Part print with two shaded views. Sizes in mm from the minimum x, y, z corner. Give positions to 0.01 mm unless a question says otherwise; leave off trailing zeros. Write each loop counter-clockwise with the first axis right and the second up, starting at its lowest first coordinate (ties: lowest second). Pieces come first, ordered by that corner, then holes. Notation, with made-up numbers: (44, 40) - (80, 40) arc R17 ccw to (80, 49) - close; hole circle Ø9 at (-9, 29.5). An arc over 180 degrees is marked (long way). Answer as a JSON object with one key per item and string values.
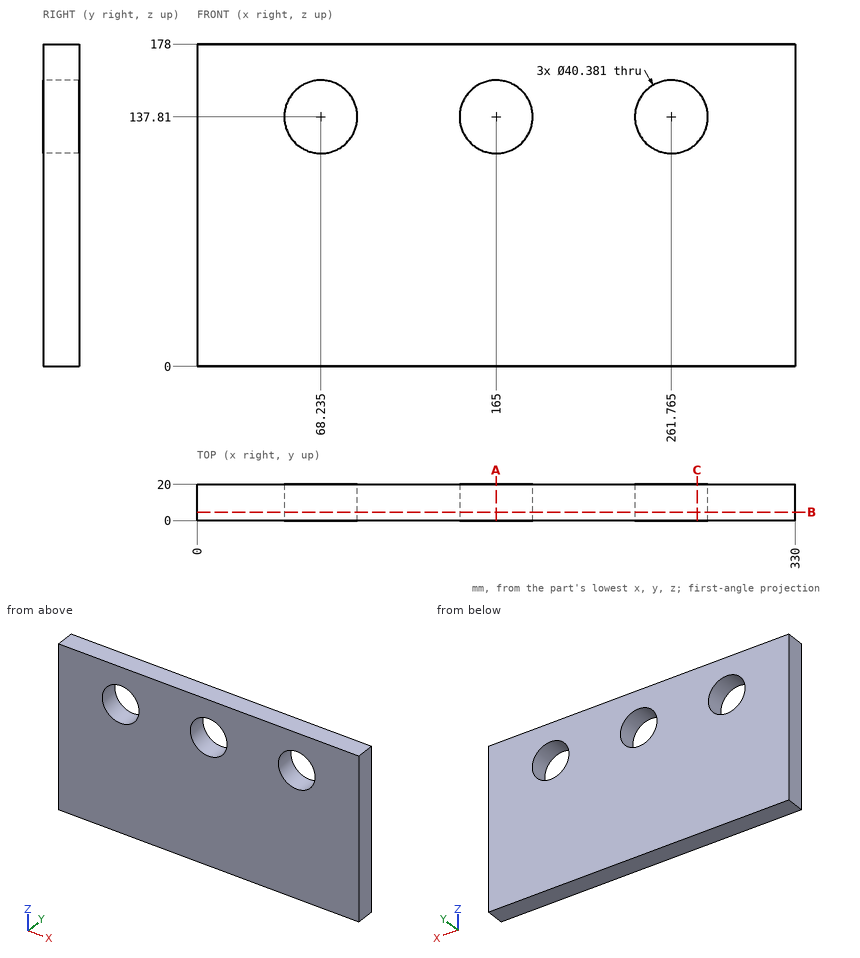
(1) Saw through at A-A, the plane x = 165. Give the cut face in (y, z), and give its area (3 significant figures).
Answer key:
{"outline": "(0, 0) - (20, 0) - (20, 117.62) - (0, 117.62) - close; (0, 158) - (20, 158) - (20, 178) - (0, 178) - close", "area": "2,750 mm²"}
(2) Probe L1, parallel to Z at x = 165, y = 12.5; L2, parallel to X at y = 1, z = 150.5 (1 decimal); L3, parallel to X at y = 9.75, z = 140 (1 decimal). List the from-to ranges inside material, lowest first. Write a range as [from, to].
Answer key:
{"L1": "z = [0, 117.62], [158, 178]", "L2": "x = [0, 52.5], [83.9, 149.3], [180.7, 246.1], [277.5, 330]", "L3": "x = [0, 48.2], [88.3, 144.9], [185.1, 241.7], [281.8, 330]"}
(3) Saw through at B-B, the plane y = 4.75. Give the cut face in (x, z) (1 decimal), and give its area (3 significant figures).
Answer key:
{"outline": "(0, 0) - (330, 0) - (330, 178) - (0, 178) - close; hole circle Ø40.4 at (68.2, 137.8); hole circle Ø40.4 at (165, 137.8); hole circle Ø40.4 at (261.8, 137.8)", "area": "54,900 mm²"}
(4) Saw through at C-C, the plane x = 276. Give the cut face in (y, z), and give its area (3 significant figures).
Answer key:
{"outline": "(0, 0) - (20, 0) - (20, 123.49) - (0, 123.49) - close; (0, 152.13) - (20, 152.13) - (20, 178) - (0, 178) - close", "area": "2,990 mm²"}
